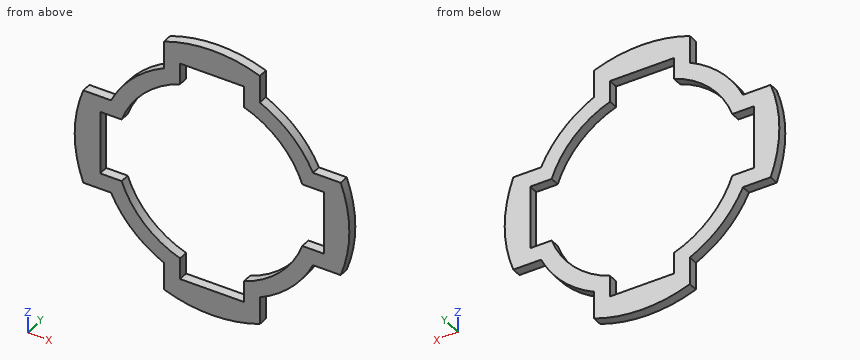
```python
from build123d import *

# Parameters (mm, degrees)
BOSS_EXTRUDE1_DEPTH = 0.3


with BuildPart() as part:
    # Sketch1 → Boss-Extrude1 (new body)
    with BuildSketch(Plane(origin=(0, 0, 0), x_dir=(1, 0, 0), z_dir=(0, 1, 0))):
        with BuildLine():
            Line((-4.029888336, 1.5), (-3.16227766, 1.5))
            ThreePointArc((-3.16227766, 1.5), (-2.474873734, 2.474873734), (-1.5, 3.16227766))
            Line((-1.5, 3.16227766), (-1.5, 4.029888336))
            ThreePointArc((-1.5, 4.029888336), (0, 4.3), (1.5, 4.029888336))
            Line((1.5, 4.029888336), (1.5, 3.16227766))
            ThreePointArc((1.5, 3.16227766), (2.474873734, 2.474873734), (3.16227766, 1.5))
            Line((3.16227766, 1.5), (4.029888336, 1.5))
            ThreePointArc((4.029888336, 1.5), (4.3, 0), (4.029888336, -1.5))
            Line((4.029888336, -1.5), (3.16227766, -1.5))
            ThreePointArc((3.16227766, -1.5), (2.474873734, -2.474873734), (1.5, -3.16227766))
            Line((1.5, -3.16227766), (1.5, -4.029888336))
            ThreePointArc((1.5, -4.029888336), (0, -4.3), (-1.5, -4.029888336))
            Line((-1.5, -4.029888336), (-1.5, -3.16227766))
            ThreePointArc((-1.5, -3.16227766), (-2.474873734, -2.474873734), (-3.16227766, -1.5))
            Line((-3.16227766, -1.5), (-4.029888336, -1.5))
            ThreePointArc((-4.029888336, -1.5), (-4.3, 0), (-4.029888336, 1.5))
        make_face()
        with BuildLine():
            Line((-3.5, 1), (-2.828427125, 1))
            ThreePointArc((-2.828427125, 1), (-2.121320344, 2.121320344), (-1, 2.828427125))
            Line((-1, 2.828427125), (-1, 3.5))
            Line((-1, 3.5), (1, 3.5))
            Line((1, 3.5), (1, 2.828427125))
            ThreePointArc((1, 2.828427125), (2.121320344, 2.121320344), (2.828427125, 1))
            Line((2.828427125, 1), (3.5, 1))
            Line((3.5, 1), (3.5, -1))
            Line((3.5, -1), (2.828427125, -1))
            ThreePointArc((2.828427125, -1), (2.121320344, -2.121320344), (1, -2.828427125))
            Line((1, -2.828427125), (1, -3.5))
            Line((1, -3.5), (-1, -3.5))
            Line((-1, -3.5), (-1, -2.828427125))
            ThreePointArc((-1, -2.828427125), (-2.121320344, -2.121320344), (-2.828427125, -1))
            Line((-2.828427125, -1), (-3.5, -1))
            Line((-3.5, -1), (-3.5, 1))
        make_face(mode=Mode.SUBTRACT)
    extrude(amount=BOSS_EXTRUDE1_DEPTH)


solid = part.part
```
The listing builds one solid part. Answer for the finished solid, in the listing's coordinates (mm). Give positions to 0.01 mm unless a question says otherwise; leave off trailing zeros. Loops run counter-clockwise (first coordinate to the right, second up) from the corner with the lowest first, then second, coordinate; pieces in that order, holes last. Notation, with made-up numbers: (-32, 31) - (-4, 31) arc R17 cw to (-4, 35) - close; hole circle Ø9 at (-8.5, -15.5). An arc over 180 degrees is marked (long way). Answer as CSV lines item,"result". Start each with the question number.
Item 1: Find the intervals of material crossed by line 1 (Z direction, x = -2.5, y = 0.25); line 2 (Z direction, x = 3.25, y = 0.1), in increasing order. Write a range as from..to.
Item 2: A cutting plane is placed at B-B on x = 2.25. Determine the outline of the cut face in (y, z).
Item 3: A cutting plane is placed at A-A on z = -2. Determine the outline of the cut face in (x, y).
Found:
1,line 1,"z = -2.45..-1.66, 1.66..2.45"
1,line 2,"z = -1.5..-1, 1..1.5"
2,outline,"(0, -2.68) - (0.3, -2.68) - (0.3, -1.98) - (0, -1.98) - close; (0, 1.98) - (0.3, 1.98) - (0.3, 2.68) - (0, 2.68) - close"
3,outline,"(-2.87, 0) - (-2.24, 0) - (-2.24, 0.3) - (-2.87, 0.3) - close; (2.24, 0) - (2.87, 0) - (2.87, 0.3) - (2.24, 0.3) - close"
